Read the model definition and answer for the solid it produces. Units are mm, in the model's axes. Face numbers are marked on the shaded views. A direction names the side the tool comes from. Give positions to 0.01 mm unless a question says otherwise; leave off trailing zeros. Loops run counter-clockwise (first coordinate to the right, second up) from the corner with the lowest first, then second, coordinate; pieces in that order, holes last. Notation, with made-up numbers: (18.25, 67) - (59.25, 67) arc R25 ccw to (59.25, 83) - close; hole circle Ø7 at (2.25, 22.5). An arc over 180 degrees is marked (long way). Put each result on its own line as item: value. Start each with the question number.
1. A cutting plane is placed at A-A, the plane x = 0.75. Determine the outline of the cut face in (y, z), plus the area to 3 significant figures.
2. A cutting plane is placed at C-C, the plane x = 6.5. Determine the outline of the cut face in (y, z), plus the area to 4 significant figures.
3. Given pin 1 Ø8 at (x, z) = (4, 8) entering from -Y; pin 2 Ø7 at (x, z) = (0, 22.7) entering from +Y; pin 3 Ø1.5 at (x, y) = (0, -6) entering from +Z, each flat-ended and moving along its own axis, determine where each tip first touches the part or whether it passes through.
4. For the marked faces 4, 5 and 6, determine the directions among +Z, -Z, +X, -X, +Y, -Y from which every point of the face is accessible in a straight line to the end or side of a thin tool.
5. A cutting plane is placed at D-D, the plane y = -0.75. Determine the outline of the cut face in (x, z), plus the area to 3 significant figures.
6. Consider L1, parallel to X at y = -2.5, z = 23.5; L2, parallel to Z at x = 0, y = -4.05; L3, parallel to X at y = -5.25, z = 17. Determine where each line is inside the solid, lowest interval first. Write a range as from..to.
7. A cutting plane is placed at B-B, the plane z = 9.25. Determine the outline of the cut face in (x, y), plus the area to 3 significant figures.
8. For a pull along Z with two mould halves and no side action, classify the marked faces 1, 2 and 3 as released by +Z, released by -Z, zero draft, split by the parting line, or undercut.
```python
from build123d import *

# Parameters (mm, degrees)
F1_DEPTH  = 0.7
F3_DEPTH  = 4
F5_DEPTH  = 9
F6_W      = 16
F6_H      = 7
F7_DEPTH  = 14
F8_R      = 2.75
F9_DEPTH  = 7.001
F10_R     = 2.75
F11_DEPTH = 2
F12_R     = 2.75
F13_DEPTH = 3
F14_SIZE2 = 0.5
F14_SIZE  = 0.2886751346


with BuildPart() as f1:
    # F0 (on Top) → F1 (new body)
    with BuildSketch(Plane.XY):
        with BuildLine():
            Line((5.657, 0), (-5.657, 0))
            ThreePointArc((-5.657, 0), (-3.4641611178, -2.8989837358), (0, -4))
            ThreePointArc((0, -4), (3.4641611178, -2.8989837358), (5.657, 0))
        make_face()
        with BuildLine():
            ThreePointArc((0, -4), (-3.4641611178, -2.8989837358), (-5.657, 0))
            Line((-5.657, 0), (-5.657, -2))
            Line((-5.657, -2), (-3.9498932188, -3.7071067812))
            ThreePointArc((-3.9498932188, -3.7071067812), (-3.62546987, -3.9238795325), (-3.2427864376, -4))
            Line((-3.2427864376, -4), (0, -4))
        make_face()
        with BuildLine():
            Line((5.657, -2), (5.657, 0))
            ThreePointArc((5.657, 0), (3.4641611178, -2.8989837358), (0, -4))
            Line((0, -4), (3.2427864376, -4))
            ThreePointArc((3.2427864376, -4), (3.62546987, -3.9238795325), (3.9498932188, -3.7071067812))
            Line((3.9498932188, -3.7071067812), (5.657, -2))
        make_face()
    extrude(amount=F1_DEPTH)

    # F2 (on face) → F3 (join)
    with BuildSketch(Plane.XY.offset(0.7)):
        with BuildLine():
            Line((5.657, 0), (-5.657, 0))
            ThreePointArc((-5.657, 0), (-3.4641611178, -2.8989837358), (0, -4))
            ThreePointArc((0, -4), (3.4641611178, -2.8989837358), (5.657, 0))
        make_face()
    extrude(amount=F3_DEPTH)

    # F4 (on face) → F5 (join)
    with BuildSketch(Plane.XY.offset(4.7)):
        with BuildLine():
            Line((5.657, 0), (-5.657, 0))
            ThreePointArc((-5.657, 0), (0, -4), (5.657, 0))
        make_face()
        with BuildLine():
            Line((-5.657, 0), (-7, 0))
            Line((-7, 0), (-7, -4))
            Line((-7, -4), (-6, -5))
            Line((-6, -5), (6, -5))
            Line((6, -5), (7, -4))
            Line((7, -4), (7, 0))
            Line((7, 0), (5.657, 0))
            ThreePointArc((5.657, 0), (0, -4), (-5.657, 0))
        make_face()
    extrude(amount=F5_DEPTH)

    # F6 (on face) → F7 (join)
    with BuildSketch(Plane.XY.offset(13.7)):
        with Locations((0, -3.5)):
            Rectangle(F6_W, F6_H)
    extrude(amount=F7_DEPTH)

    # F8 (on face) → F9 (cut, through all)
    with BuildSketch(Plane.XZ.offset(7)):
        with Locations((0, 22.7)):
            Circle(F8_R)
    extrude(amount=-F9_DEPTH, mode=Mode.SUBTRACT)

    # F10 (on face) → F11 (cut)
    with BuildSketch(Plane.XZ.offset(7)):
        with BuildLine():
            Line((6, 27.7), (-6, 27.7))
            Line((-6, 27.7), (-6, 17.7))
            ThreePointArc((-6, 17.7), (-4, 15.7), (-2, 17.7))
            Line((-2, 17.7), (2, 17.7))
            ThreePointArc((2, 17.7), (4, 15.7), (6, 17.7))
            Line((6, 17.7), (6, 27.7))
        make_face()
        with Locations((0, 22.7)):
            Circle(F10_R, mode=Mode.SUBTRACT)
    extrude(amount=-F11_DEPTH, mode=Mode.SUBTRACT)

    # F12 (on face) → F13 (cut)
    with BuildSketch(Plane(origin=(0, 0, 0), x_dir=(-1, 0, 0), z_dir=(0, 1, 0))):
        with BuildLine():
            Line((5, 27.7), (-5, 27.7))
            Line((-5, 27.7), (-5, 22.7))
            ThreePointArc((-5, 22.7), (0, 17.7), (5, 22.7))
            Line((5, 22.7), (5, 27.7))
        make_face()
        with Locations((0, 22.7)):
            Circle(F12_R, mode=Mode.SUBTRACT)
    extrude(amount=-F13_DEPTH, mode=Mode.SUBTRACT)

    # F14
    f14_edges = [f1.edges().sort_by_distance(p)[0] for p in [
        (0, 0, 0),
        (-5.657, -1, 0),
        (-4.803447, -2.853553, 0),
        (-3.62547, -3.92388, 0),
        (0, -4, 0),
        (3.62547, -3.92388, 0),
        (4.803447, -2.853553, 0),
        (5.657, -1, 0),
    ]]
    f14_side = f1.faces().sort_by_distance((0, -1.868566, 0))[0]
    chamfer(f14_edges, length=F14_SIZE, length2=F14_SIZE2, reference=f14_side)


solid = f1.part
```
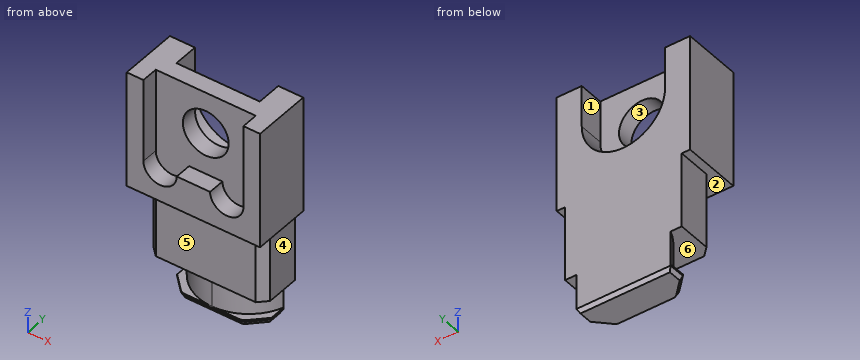
Return value:
1. outline: (-7, 13.7) - (-5, 13.7) - (-5, 4.7) - (-3.95, 4.7) - (-3.95, 0.7) - (-4, 0.7) - (-4, 0.5) - (-3.71, 0) - (-0.29, 0) - (0, 0.5) - (0, 17.76) - (-3, 17.76) - (-3, 20.05) - (-5, 20.05) - (-5, 17.7) - (-7, 17.7) - close; (-5, 25.35) - (-3, 25.35) - (-3, 27.7) - (-5, 27.7) - close
1. area: 101 mm2
2. outline: (-7, 13.7) - (-4.5, 13.7) - (-4.5, 4.7) - (0, 4.7) - (0, 27.7) - (-7, 27.7) - close
2. area: 138.5 mm2
3. pin 1: stops at y = -5
3. pin 2: stops at y = -3
3. pin 3: stops at z = 17.7
4. face 4: -Z, +X, +Y, -Y
4. face 5: -Z, +X, -X, -Y
4. face 6: -Y
5. outline: (-8, 13.7) - (-7, 13.7) - (-7, 4.7) - (-5.33, 4.7) - (-5.33, 0.7) - (-5.66, 0.7) - (-5.66, 0.5) - (-5.37, 0) - (5.37, 0) - (5.66, 0.5) - (5.66, 0.7) - (5.33, 0.7) - (5.33, 4.7) - (7, 4.7) - (7, 13.7) - (8, 13.7) - (8, 27.7) - (5, 27.7) - (5, 22.7) arc R5 cw to (-5, 22.7) - (-5, 27.7) - (-8, 27.7) - close
5. area: 311 mm2
6. L1: x = -8..-5, 5..8
6. L2: z = 4.7..19.95, 25.45..27.7
6. L3: x = -8..-5.87, -2.13..2.13, 5.87..8
7. outline: (-7, -4) - (-6, -5) - (6, -5) - (7, -4) - (7, 0) - (-7, 0) - close
7. area: 69.0 mm2
8. face 1: zero draft
8. face 2: released by -Z
8. face 3: undercut
